Geometry check sheet. Reference: drawing and pictorial views, mm from the part's lowest x, y, z. Give positions to 0.01 mm unless a question says otherwise; leave off trailing zeros. Order: outer loops, then holes, each group sorted by start corner. A loop starts at its lowest first (then second) coordinate and runs counter-clockwise, first axis right, second up.
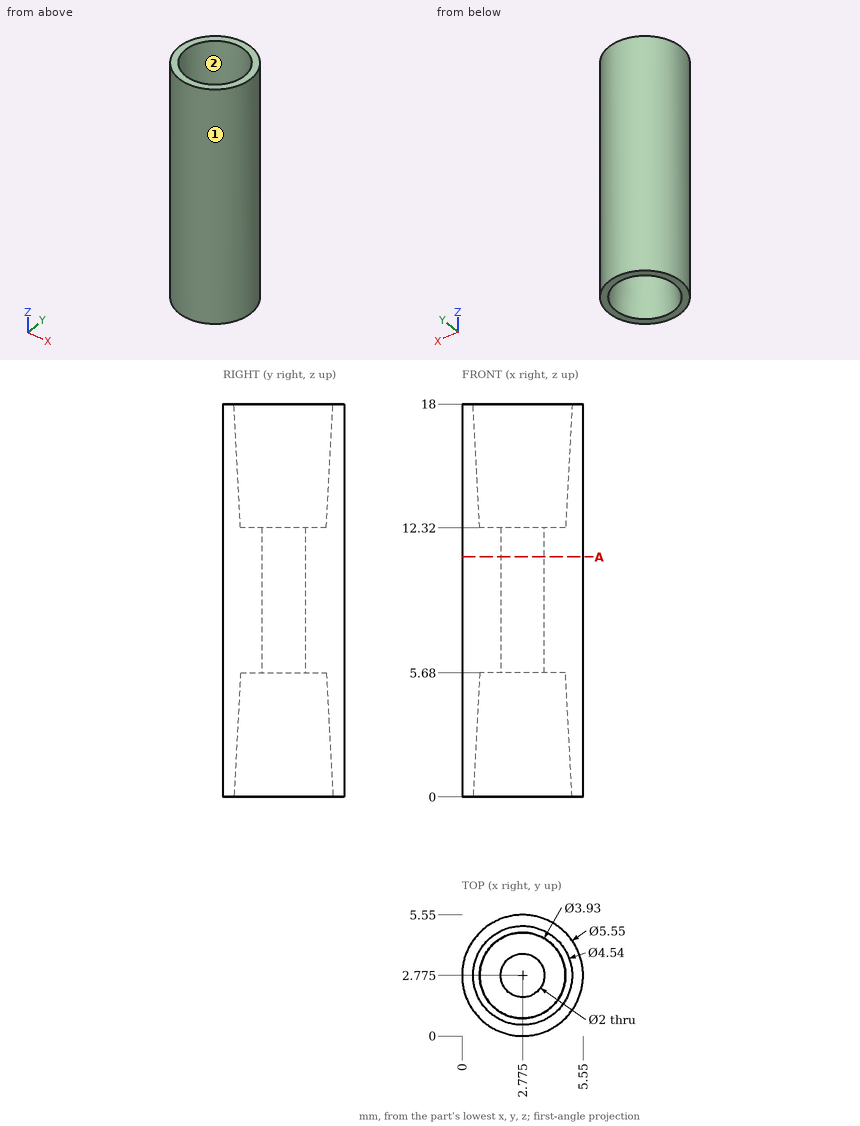
(1) Thickness scan on L1, parallel to Y at x = 4.6, z = 1 (1 decimal); L2, parallel to X at y = 3.65, z = 1.25; L3, parallel to Y at x = 2.55, z = 6.5. Record the ranges inside material, lowest first.
(2) Go/stop test with flat-tipped pins: P1, Ø1.6, axis at x = 2.775, y = 2.775, coming from the -Z side; P2, Ø1.5, axis at x = 3.5, y = 3, coming from the -Z side; P3, Ø2, axis at x = 2, y = 3, coming from the +Z side. Record where each tip stops, or that it passes through.
(3) Sectioned sample at A-A (z = 11). Enter the section's corners in (x, y) (3 decimals), plus the area to 4 significant figures.
(4) Release check for a two-part mould opening along X. For the marked faces 1 and 2 record: released by +X, released by -X, zero draft, split by the parting line, or undercut.
Values follow:
1. L1: y = 0.7 to 1.5, 4 to 4.9
1. L2: x = 0.14 to 0.75, 4.8 to 5.41
1. L3: y = 0.01 to 1.8, 3.75 to 5.54
2. P1: passes through
2. P2: stops at z = 5.68
2. P3: stops at z = 12.32
3. outline: circle Ø5.55 at (2.775, 2.775); hole circle Ø2 at (2.775, 2.775)
3. area: 21.05 mm2
4. face 1: split by the parting line
4. face 2: undercut
